Read the model definition and answer for the solid it produces. Units are mm, in the model's axes. Face numbers are marked on the shaded views. A direction names the side the tool comes from. Round coordinates to 2 decimals unless told otherwise and drop trailing zeros. Write each loop counter-clockwise with the first axis right and the second up, starting at its lowest first coordinate (ties: lowest second). Pieces come first, ordered by that corner, then holes.
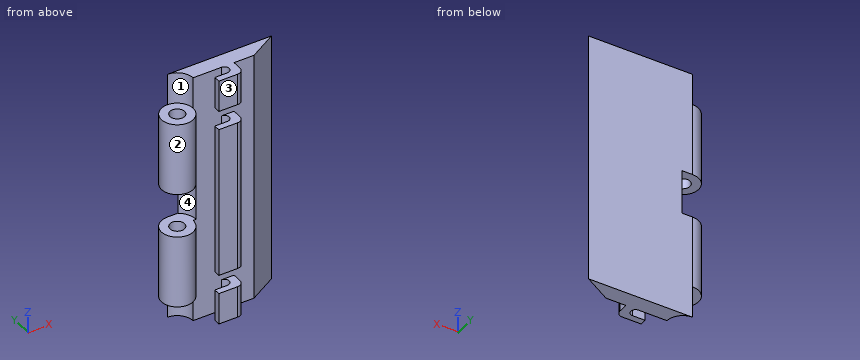
from build123d import *

# Parameters (mm, degrees)
SKETCH_1_R          = 1.15
EXTRUDE_1_DEPTH     = 20
EXTRUDE_2_DEPTH     = 20
SKETCH_5_R          = 3
CUT_EXTRUDE_2_DEPTH = 3.5
CUT_EXTRUDE_START   = -5
SKETCH_6_R          = 2.5
CUT_EXTRUDE_3_DEPTH = 5
SKETCH_7_R          = 2.5
CUT_EXTRUDE_4_DEPTH = 5
SKETCH_10_W         = 9.669872981
SKETCH_10_H         = 3
CUT_EXTRUDE_5_DEPTH = 3


with BuildPart() as part:
    # 草图1 → 凸台-拉伸1 (new, symmetric)
    with BuildSketch(Plane.XY):
        with BuildLine():
            Line((2.5, 0), (12.169872981, 0))
            Line((12.169872981, 0), (16.5, 2.5))
            Line((16.5, 2.5), (0, 2.5))
            ThreePointArc((0, 2.5), (-1.767766953, -1.767766953), (2.5, 0))
        make_face()
        Circle(SKETCH_1_R, mode=Mode.SUBTRACT)
    extrude(amount=EXTRUDE_1_DEPTH, both=True)

    # 草图4 → 凸台-拉伸2 (add, symmetric)
    with BuildSketch(Plane.XY):
        with BuildLine():
            Line((7, -1.5), (5, -1.5))
            Line((5, -1.5), (5, -2.5))
            Line((5, -2.5), (8, -2.5))
            ThreePointArc((8, -2.5), (8.707106781, -2.207106781), (9, -1.5))
            Line((9, -1.5), (9, 0))
            Line((9, 0), (7, 0))
            ThreePointArc((7, 0), (7.75, -0.75), (7, -1.5))
        make_face()
    extrude(amount=EXTRUDE_2_DEPTH, both=True)

    # 草图5 → 切除-拉伸2 (cut, symmetric)
    with BuildSketch(Plane.XY):
        Circle(SKETCH_5_R)
    extrude(amount=CUT_EXTRUDE_2_DEPTH, both=True, mode=Mode.SUBTRACT)

    # 草图6 → 切除-拉伸3 (cut)
    with BuildSketch(Plane(origin=(0, 0, -20), x_dir=(-1, 0, 0), z_dir=(0, 0, -1)).offset(CUT_EXTRUDE_START)):
        Circle(SKETCH_6_R)
    extrude(amount=CUT_EXTRUDE_3_DEPTH, mode=Mode.SUBTRACT)

    # 草图7 → 切除-拉伸4 (cut)
    with BuildSketch(Plane.XY.offset(20)):
        Circle(SKETCH_7_R)
    extrude(amount=-CUT_EXTRUDE_4_DEPTH, mode=Mode.SUBTRACT)

    # 草图10 → 切除-拉伸5 (cut)
    with BuildSketch(Plane.XZ):
        with Locations((7.334936491, -13.5)):
            Rectangle(SKETCH_10_W, SKETCH_10_H)
        with Locations((7.334936491, 13.5)):
            Rectangle(SKETCH_10_W, SKETCH_10_H)
    extrude(amount=CUT_EXTRUDE_5_DEPTH, mode=Mode.SUBTRACT)


solid = part.part
Q1. Straight lines are drawn through the part: probe 1 along Z at (x, y) = (2.5, 0.9); probe 2 along Y at (x, z) = (0, -8.5); probe 3 along Z at (x, y) = (1.5, 0.9). For each, find the intervals that lie inside material, in ascending order.
Verdict:
probe 1: z = -20 to -3.5, 3.5 to 20
probe 2: y = -2.5 to -1.15, 1.15 to 2.5
probe 3: z = -15 to -3.5, 3.5 to 15
Q2. Flat-ended cylindrical pins translate along their axes: pin 1 Ø1.5 at (y, z) = (-1.5, -15.5) entering from +X; pin 2 Ø1.5 at (x, y) = (-1, -1) entering from -Z; pin 3 Ø0.5 at (y, z) = (-2, -16.5) entering from -X. Find the tip coordinate at first contact, or state that the pin passes through.
Verdict:
pin 1: stops at x = 9
pin 2: stops at z = -15
pin 3: stops at x = 5
Q3. Section A-A (x = 6.25) is taken. Determine the outline of the cut face in (y, z), then the cut area to 3 significant figures.
Verdict:
outline: (-2.5, -20) - (-1.5, -20) - (-1.5, -15) - (-2.5, -15) - close; (-2.5, -12) - (-1.5, -12) - (-1.5, 12) - (-2.5, 12) - close; (-2.5, 15) - (-1.5, 15) - (-1.5, 20) - (-2.5, 20) - close; (0, -20) - (2.5, -20) - (2.5, 20) - (0, 20) - close
area: 134 mm2
Q4. Section B-B (y = -0.75) is taken. Determine the outline of the cut face in (x, z).
Verdict:
outline: (-2.38, -15) - (-0.87, -15) - (-0.87, -3.5) - (-2.38, -3.5) - close; (-2.38, 3.5) - (-0.87, 3.5) - (-0.87, 15) - (-2.38, 15) - close; (0.87, -15) - (2.38, -15) - (2.38, -3.5) - (0.87, -3.5) - close; (0.87, 3.5) - (2.38, 3.5) - (2.38, 15) - (0.87, 15) - close; (7.75, -20) - (9, -20) - (9, -15) - (7.75, -15) - close; (7.75, -12) - (9, -12) - (9, 12) - (7.75, 12) - close; (7.75, 15) - (9, 15) - (9, 20) - (7.75, 20) - close
Q5. Determine the mould class of the marked faces 3 and 4 for opening direction Z: pulls with the +Z half, pulls with the -Z half, needs draft (parallel to the pull), parting line crosses it, or undercut.
Verdict:
face 3: needs draft
face 4: undercut
Q6. Section C-C (z = -14) is taken. Determine the outline of the cut face in (x, y), then the cut area to 3 significant figures.
Verdict:
outline: (0, 2.5) arc R2.5 ccw (long way) to (2.5, 0) - (12.17, 0) - (16.5, 2.5) - close; hole circle Ø2.3 at (0, 0)
area: 46.4 mm2
Q7. Section D-D (x = -0.5) is taken. Determine the outline of the cut face in (y, z).
Verdict:
outline: (-2.45, -15) - (-1.04, -15) - (-1.04, -3.5) - (-2.45, -3.5) - close; (-2.45, 3.5) - (-1.04, 3.5) - (-1.04, 15) - (-2.45, 15) - close; (1.04, -15) - (2.45, -15) - (2.45, -3.5) - (1.04, -3.5) - close; (1.04, 3.5) - (2.45, 3.5) - (2.45, 15) - (1.04, 15) - close
Q8. Which of the six approach directions +Z, -Z, +X, -X, +Y, -Y give full straight-line access (tool end or side, diameter ignored) to the marked faces 1 and 2?
Verdict:
face 1: +Z, -X, -Y
face 2: +Z, -Z
